Design review of the part built by this model. Coordinates are the model's own, in mm. Face numbers are marked on the shaded views. A direction names the side the tool comes from. Round coordinates to 2 decimals unless told otherwise and drop trailing zeros. Write each loop counter-clockwise with the first axis right and the second up, starting at its lowest first coordinate (ties: lowest second). Pieces come first, ordered by that corner, then holes. Notation, with made-up numbers: M 21,1.25 L 61,1.25 A6 ccw 61,7.25 Z; hole C 14,-0.5 d1. An arc over 180 degrees is marked long. One line per question, with ' | ' between items. Start each with the question number.
Item 1: Draft analysis for pull direction Y (two halves, no side actions). For the marked faces 3, 4 and 5, state which applies: released by +Y, released by -Y, zero draft, split by the parting line, or undercut.
Item 2: Insertion check: pin 1 Ø7.5 at (x, z) = (41.28, 14.41) entering from +Y. The pin has a flat end and moves straight along its axis. Give the tip position at first contact, or say it passes through.
Item 3: Add section A-A, the plane y = -33.5. State the section outline as (x, z) points, and give its area (3 significant figures).
Item 4: Add section C-C, the plane z = 25.75. State the section outline as (x, y) points.
Item 5: For L1, parallel to X at y = -34, z = 22.25, list the stretches that pass through material, from the lowest coordinate up.
Item 6: Add section D-D, the plane x = -38. State the section outline as (y, z) points.
Item 7: Machinability: for the marked faces 1 and 2, which of the approach directions +Z, -Z, +X, -X, +Y, -Y give a long, thin tool a straight path to every point of the face, cutting with its end or side? Answer none if there is none.
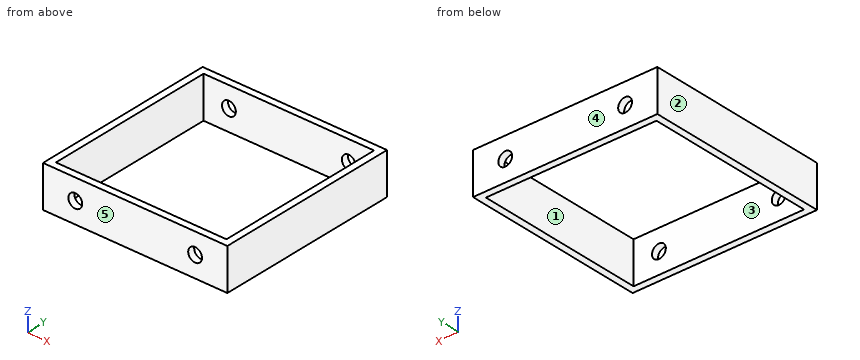
```python
from build123d import *

# Parameters (mm, degrees)
SKETCH2_W           = 127
SKETCH2_H           = 127
BOSS_EXTRUDE1_DEPTH = 28.702
SKETCH3_W           = 117.475
SKETCH3_H           = 117.475
CUT_EXTRUDE1_DEPTH  = 28.702
CUT_EXTRUDE2_REACH  = 146.862
SKETCH4_R           = 4.7625


with BuildPart() as part:
    # Sketch2 → Boss-Extrude1 (new body)
    with BuildSketch(Plane.XY):
        Rectangle(SKETCH2_W, SKETCH2_H)
    extrude(amount=BOSS_EXTRUDE1_DEPTH)

    # Sketch3 → Cut-Extrude1 (cut)
    with BuildSketch(Plane.XY.offset(28.702)):
        Rectangle(SKETCH3_W, SKETCH3_H)
    extrude(amount=-CUT_EXTRUDE1_DEPTH, mode=Mode.SUBTRACT)

    # Cut-Extrude2: up to this face of the body (flat: up to its plane)
    cut_extrude2_end = Plane(part.part.faces().sort_by_distance((0, -63.5, 14.351))[0])
    # Sketch4 → Cut-Extrude2 (cut, up to the picked face)
    with BuildSketch(Plane(origin=(0, 63.5, 0), x_dir=(1, 0, 0), z_dir=(0, 1, 0)), mode=Mode.PRIVATE) as cut_extrude2_sk1:
        with Locations(Location((41.275, -14.4145, 0), (0, 0, 270))):
            Circle(SKETCH4_R)
    cut_extrude2_tool1 = split(extrude(cut_extrude2_sk1.sketch, amount=-CUT_EXTRUDE2_REACH, mode=Mode.PRIVATE), bisect_by=cut_extrude2_end, keep=Keep.BOTH, mode=Mode.PRIVATE)
    # Sketch4 → Cut-Extrude2 (cut, up to the picked face)
    with BuildSketch(Plane(origin=(0, 63.5, 0), x_dir=(1, 0, 0), z_dir=(0, 1, 0)), mode=Mode.PRIVATE) as cut_extrude2_sk2:
        with Locations(Location((-41.275, -14.4145, 0), (0, 0, 270))):
            Circle(SKETCH4_R)
    cut_extrude2_tool2 = split(extrude(cut_extrude2_sk2.sketch, amount=-CUT_EXTRUDE2_REACH, mode=Mode.PRIVATE), bisect_by=cut_extrude2_end, keep=Keep.BOTH, mode=Mode.PRIVATE)
    add(cut_extrude2_tool1.solids().sort_by(Axis((41.275, 63.5, 14.4145), (0, -1, 0)))[0], mode=Mode.SUBTRACT)
    add(cut_extrude2_tool2.solids().sort_by(Axis((-41.275, 63.5, 14.4145), (0, -1, 0)))[0], mode=Mode.SUBTRACT)


solid = part.part
```
Computed values:
1) face 3: undercut | face 4: released by +Y | face 5: released by -Y
2) pin 1: passes through
3) outline: M -63.5,0 L -58.74,0 L -58.74,28.7 L -63.5,28.7 Z; M 58.74,0 L 63.5,0 L 63.5,28.7 L 58.74,28.7 Z | area: 273 mm^2
4) outline: M -63.5,-63.5 L 63.5,-63.5 L 63.5,63.5 L -63.5,63.5 Z; hole M -58.74,-58.74 L 58.74,-58.74 L 58.74,58.74 L -58.74,58.74 Z
5) L1: x = -63.5 to -58.74, 58.74 to 63.5
6) outline: M -63.5,0 L -58.74,0 L -58.74,10.96 L -63.5,10.96 Z; M -63.5,17.87 L -58.74,17.87 L -58.74,28.7 L -63.5,28.7 Z; M 58.74,0 L 63.5,0 L 63.5,10.96 L 58.74,10.96 Z; M 58.74,17.87 L 63.5,17.87 L 63.5,28.7 L 58.74,28.7 Z
7) face 1: +Z, -Z | face 2: +Z, -Z, -X, +Y, -Y
